Could you check a few things on this model? Use its own coordinates, in mm. Face numbers are marked on the shaded views. A direction names the side the tool comes from. Give positions to 0.01 mm unless a question says otherwise; leave off trailing zeros. Order: outer loops, then holes, each group sorted by start corner. A loop starts at its lowest first (then second) coordinate and runs counter-clockwise, first axis right, second up. Notation, with made-up numbers: M -6,71 L 26,71 A17 cw 26,82 Z; hole C 87,29.5 d11. An arc over 180 degrees is marked long. Use a Markdown table: item, result. Add a question column.
```python
from build123d import *

# Parameters (mm, degrees)
F1_DEPTH       = 60
F3_D           = 4
F3_CSINK_D     = 9
F3_CSINK_ANGLE = 90
F4_C1_SIZE2    = 1.6076951546
F4_C1_SIZE     = 6
F4_C2_SIZE2    = 6
F4_C2_SIZE     = 1.6076951546
F6_R           = 10
F5_W           = 8
F5_H           = 10
F7_DEPTH       = 10
F8_SIZE        = 8
F10_DEPTH      = 9.7
F11_SIZE2      = 1.9395967878
F11_SIZE       = 11


# Not quite as in the source:
# - a feature names something its author has since deleted; it is built from what else it names


with BuildPart() as f1:
    # F0 (on Top) → F1 (new body)
    with BuildSketch(Plane.XY):
        Polygon((4.85, 0), (27.5, 0), (27.5, 5), (-27.5, 5), (-27.5, 0), (-4.85, 0), (-4.85, -8), (4.85, -8), align=None)
    extrude(amount=F1_DEPTH)

    # F3 (through all)
    with Locations(Plane.XZ):
        with Locations((-12.5, 50), (-12.5, 25), (12.5, 50), (12.5, 25)):
            CounterSinkHole(F3_D / 2, F3_CSINK_D / 2, counter_sink_angle=F3_CSINK_ANGLE)

    # F4: chamfer of 6 x 1.6076951546 on 2 edges, made by hand

    # F4_c1
    f4_c1_edges = [f1.edges().sort_by_distance(p)[0] for p in [
        (4.85, -4, 0),
    ]]
    f4_c1_side = f1.faces().sort_by_distance((4.85, -4, 0.0321539031))[0]
    chamfer(f4_c1_edges, length=F4_C1_SIZE, length2=F4_C1_SIZE2, reference=f4_c1_side)

    # F4_c2
    f4_c2_edges = [f1.edges().sort_by_distance(p)[0] for p in [
        (-4.85, -4, 0),
    ]]
    f4_c2_side = f1.faces().sort_by_distance((-4.8178460969, -4, 0))[0]
    chamfer(f4_c2_edges, length=F4_C2_SIZE, length2=F4_C2_SIZE2, reference=f4_c2_side)

    # F6
    f6_edges = [f1.edges().sort_by_distance(p)[0] for p in [
        (-4.85, -4, 6),
        (4.85, -4, 6),
    ]]
    fillet(f6_edges, radius=F6_R)

    # F5 (on face) → F7 (join)
    with BuildSketch(Plane.XZ):
        with Locations((-23.5, 50)):
            Rectangle(F5_W, F5_H)
        with Locations((23.5, 50)):
            Rectangle(F5_W, F5_H)
    extrude(amount=F7_DEPTH)

    # F8
    f8_edges = [f1.edges().sort_by_distance(p)[0] for p in [
        (-23.5, -10, 55),
        (23.5, -10, 55),
    ]]
    chamfer(f8_edges, length=F8_SIZE)

    # F9 (on face) → F10 (cut, through all)
    with BuildSketch(Plane.YZ.offset(4.85)):
        Polygon((0, 51.0882381259), (-8, 54), (-8, 19.3165249759), (0, 22.22828685), align=None)
    extrude(amount=-F10_DEPTH, mode=Mode.SUBTRACT)

    # F11
    f11_edges = [f1.edges().sort_by_distance(p)[0] for p in [
        (0, -8, 0),
    ]]
    f11_side = f1.faces().sort_by_distance((0, -8, 10.07737))[0]
    chamfer(f11_edges, length=F11_SIZE, length2=F11_SIZE2, reference=f11_side)


solid = f1.part
```
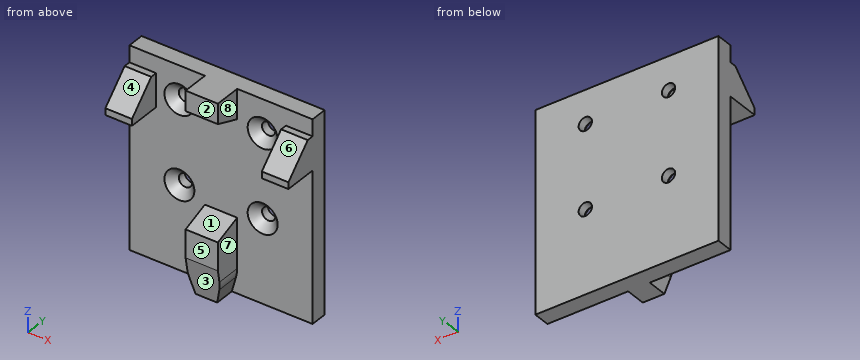
1) Suppose I cut it at A-A on z = 25. Please give me the cut outline in (x, y), and give its area (4 significant figures).
2) Suppose I cut it at D-D on z = 6. Please give me the cut outline in (x, y), and give its area (3 significant figures).
3) Suppose I cut it at C-C on y = -3.5. Please give me the cut outline in (x, z), and give its area (3 significant figures).
4) For the marked faces 5, 6, 7 and 8, which set-ups out of +Z, -Z, +X, -X, +Y, -Y let a thin tool reach every point of the face, with its end or its side?
5) We'd pull the mould along Z, two halves only. Please class the marked faces 1, 2, 3 and 4: pulls with the +Z half, pulls with the -Z half, needs draft (parallel to the pull), parting line crosses it, or undercut.
6) For pin 1 (4 mm diameter, centred on x = -25.5, y = -7, fed in from -Z); pin 2 (4 mm diameter, centred on y = -5, z = 18, fed in from +X); pin 3 (2.5 mm diameter, centred on x = 1.5, z = 15.5, fed in from -Y), each with a flat end and sliding along its axis, tell me the tip position at first contact or that it passes through.
7) Please list where these lines run through material, in increasing order: line 1 (Z direction, x = 12.5, y = 3.6); line 2 (X direction, y = 3.5, z = 25); line 3 (X direction, y = -6.5, z = 46.5). Write a range as from..to.
8) Suppose I cut it at B-B on x = 12.5. Please give me the cut outline in (y, z), and give its area (4 significant figures).
Values found:
| question | item | result |
|---|---|---|
| 1 | outline | M -27.5,0 L -17,0 L -14.5,2.5 L -14.5,5 L -27.5,5 Z; M -10.5,2.5 L -8,0 L 8,0 L 10.5,2.5 L 10.5,5 L -10.5,5 Z; M 14.5,2.5 L 17,0 L 27.5,0 L 27.5,5 L 14.5,5 Z |
| 1 | area | 222.5 mm^2 |
| 2 | outline | M -27.5,0 L -4.76,0 L -4.76,-7.12 L 4.76,-7.12 L 4.76,0 L 27.5,0 L 27.5,5 L -27.5,5 Z |
| 2 | area | 343 mm^2 |
| 3 | outline | M -27.5,45 L -19.5,45 L -19.5,53.5 L -27.5,53.5 Z; M -4.85,7.32 A10 ccw -4.51,4.73 L -3.24,0 L 3.24,0 L 4.51,4.73 A10 ccw 4.85,7.32 L 4.85,20.95 L -4.85,20.95 Z; M -4.85,52.36 L 4.85,52.36 L 4.85,60 L -4.85,60 Z; M 19.5,45 L 27.5,45 L 27.5,53.5 L 19.5,53.5 Z |
| 3 | area | 404 mm^2 |
| 4 | face 5 | +Z, -Z, +X, -X, -Y |
| 4 | face 6 | +Z, +X, -Y |
| 4 | face 7 | +Z, -Z, +X, -Y |
| 4 | face 8 | +Z, -Z, -Y |
| 5 | face 1 | undercut |
| 5 | face 2 | needs draft |
| 5 | face 3 | pulls with the -Z half |
| 5 | face 4 | pulls with the +Z half |
| 6 | pin 1 | stops at z = 45 |
| 6 | pin 2 | stops at x = 4.85 |
| 6 | pin 3 | stops at y = -8 |
| 7 | line 1 | z = 0..23, 27..48, 52..60 |
| 7 | line 2 | x = -27.5..-14.5, -10.5..10.5, 14.5..27.5 |
| 7 | line 3 | x = -27.5..-19.5, 19.5..27.5 |
| 8 | outline | M 0,0 L 5,0 L 5,23 L 2.5,23 L 0,20.5 Z; M 0,29.5 L 2.5,27 L 5,27 L 5,48 L 2.5,48 L 0,45.5 Z; M 0,54.5 L 2.5,52 L 5,52 L 5,60 L 0,60 Z |
| 8 | area | 247.5 mm^2 |
